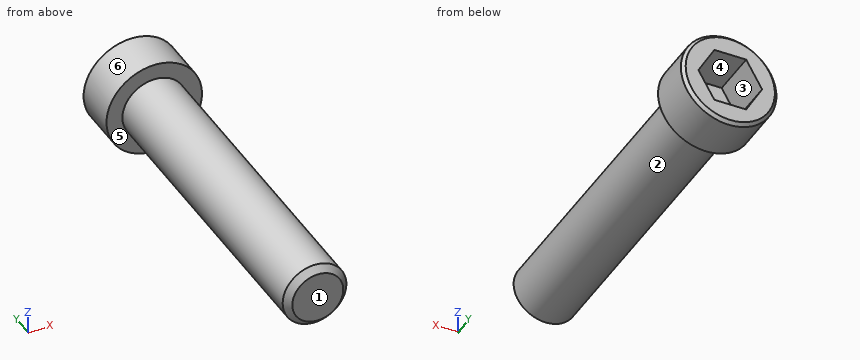
Autodesk Inventor part; units mm, degrees
ref_plane "YZ Plane" through (0, 0, 0) normal (1, 0, 0) x (0, 1, 0)
ref_plane "XZ Plane" through (0, 0, 0) normal (0, 1, 0) x (-1, 0, 0)
ref_plane "XY Plane" through (0, 0, 0) normal (0, 0, 1) x (1, 0, 0)
sketch "Sketch1" plane through (0, 0, 0) normal (0, 1, 0) x (-1, 0, 0)
  circle A0 centre (0, 0) radius 1
  dimension "d0" = 2
extrude "Extrusion1" add sketch "Sketch1" along normal blind 10
sketch "Sketch2" plane through (0, 10, 0) normal (0, 1, 0) x (1, 0, 0)
  circle A0 centre (0, 0) radius 1.5
  dimension "d3" = 3
extrude "Extrusion2" add sketch "Sketch2" along normal blind 1.5
sketch "Sketch3" plane through (0, 11.5, 0) normal (0, 1, 0) x (1, 0, 0)
  circle A0 centre (0, 0) radius 1
  line L0 (-1, 0) -> (-0.5, 0.866)
  line L1 (-0.5, 0.866) -> (0.5, 0.866)
  line L2 (0.5, 0.866) -> (1, 0)
  line L3 (1, 0) -> (0.5, -0.866)
  line L4 (0.5, -0.866) -> (-0.5, -0.866)
  line L5 (-0.5, -0.866) -> (-1, 0)
extrude "Extrusion3" cut sketch "Sketch3" against normal blind 1.5 contours L3 L4 L5 L0 L1 L2
chamfer "Chamfer1" distance 0.2 angle 45 1 edges at (1, 0, 0)
chamfer "Chamfer2" distance 0.1 angle 45 1 edges at (-1.5, 11.5, 0)
thread "Thread1"
properties part number "LCD Screw" material "Stainless Steel"
For this review, take the finished solid that the model builds, in its own axes (mm). Face numbers are marked on the shaded views. A direction names the side the tool comes from. Round coordinates to 2 decimals unless told otherwise and drop trailing zeros. Write each loop counter-clockwise with the first axis right and the second up, starting at its lowest first coordinate (ties: lowest second). Pieces come first, ordered by that corner, then holes. Notation, with made-up numbers: M 12,-21.75 L 19,-21.75 A11 ccw 19,-14.75 Z; hole C 6,2.25 d9. An arc over 180 degrees is marked long. One line per item, written item: value. Start each with the question number.
(1) Machinability: for the marked faces 4, 5 and 6, which of the approach directions +Z, -Z, +X, -X, +Y, -Y give a long, thin tool a straight path to every point of the face, cutting with its end or side? Answer none if there is none.
(2) The part is to be moulded in two halves that separate along X. For the marked faces 1, 2 and 3, say which applies: released by +X, released by -X, zero draft, split by the parting line, or undercut.
(3) Insertion check: pin 1 (1 mm diameter, centred on x = 0.5, y = 3, fed in from +Z). The pin has a flat end and moves straight along its axis. Give the tip position at first contact, or say it passes through.
(4) Wall thickness on line 1 (Z direction, x = 0.05, y = 5.75); line 2 (Y direction, x = -0.45, z = -1.25); line 3 (Y direction, x = -0.05, z = -0.2): over which ranges is each line inside the solid? List them lowest first.
(5) We need section A-A (x = 0). Give the boundary of the cut face in (y, z).
(6) We need section B-B (y = 3.25). Give the boundary of the cut face in (x, z).
Result:
1. face 4: +Y
1. face 5: -Y
1. face 6: +Y, -Y
2. face 1: zero draft
2. face 2: split by the parting line
2. face 3: undercut
3. pin 1: z = 1
4. line 1: -1 to 1
4. line 2: 10 to 11.5
4. line 3: 0 to 10
5. outline: M 0,-0.8 L 0.2,-1 L 10,-1 L 10,-1.5 L 11.4,-1.5 L 11.5,-1.4 L 11.5,-0.87 L 10,-0.87 L 10,0.87 L 11.5,0.87 L 11.5,1.4 L 11.4,1.5 L 10,1.5 L 10,1 L 0.2,1 L 0,0.8 Z
6. outline: C 0,0 d2
